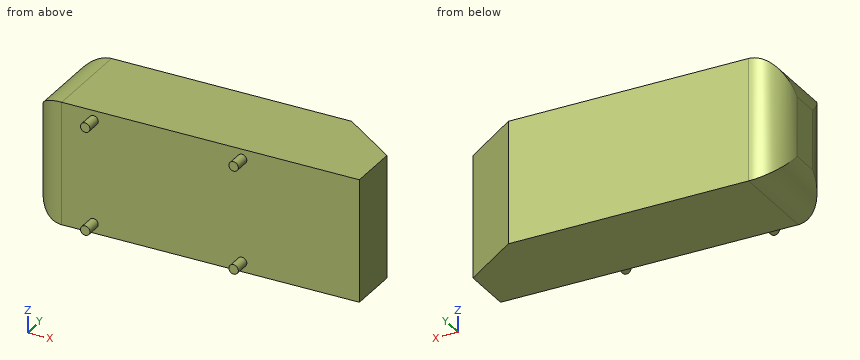
from build123d import *

# Parameters (mm, degrees)
F1_DEPTH = 194.5
F2_DEPTH = 194.5
F3_R     = 15
F5_R     = 100


with BuildPart() as f1:
    # F0 (on Top) → F1 (new body)
    with BuildSketch(Plane.XY):
        Polygon((-1043.9980842894, 48), (0, 50), (0, 210.6660311301), (-181.8517538322, 338), (-1043.9980842894, 338), (-1043.9980842894, 50), align=None)
    extrude(amount=F1_DEPTH)

    # F0 (on Top) → F2 (join)
    with BuildSketch(Plane.XY):
        Polygon((-1043.9980842894, 48), (0, 50), (0, 210.6660311301), (-181.8517538322, 338), (-1043.9980842894, 338), (-1043.9980842894, 50), align=None)
    extrude(amount=-F2_DEPTH)

    # F3 (on Front) → F4 (join, up to the next surface of F1)
    with BuildSketch(Plane.XZ):
        with Locations((-843, 163.5)):
            Circle(F3_R)
        with Locations((-843, -163.5)):
            Circle(F3_R)
        with Locations((-372, 163.5)):
            Circle(F3_R)
        with Locations((-372, -163.5)):
            Circle(F3_R)
    extrude(until=Until.NEXT, dir=(0, 1, 0))

    # F5
    f5_edges = [f1.edges().sort_by_distance(p)[0] for p in [
        (-1043.998084, 338, 0),
        (-1043.998084, 193, 194.5),
        (-1043.998084, 48, 0),
        (-1043.998084, 193, -194.5),
    ]]
    fillet(f5_edges, radius=F5_R)


solid = f1.part
CAD build for the part. Positions are in the model's coordinates, mm. Give positions to 0.01 mm unless a question says otherwise; leave off trailing zeros. Loops run counter-clockwise (first coordinate to the right, second up) from the corner with the lowest first, then second, coordinate; pieces in that order, holes last. Notation, with made-up numbers: M 85,0 L 90,0 A11 ccw 90,20 Z; hole C 53.5,19.5 d6. An arc over 180 degrees is marked long. One line per question, with ' | ' between items. Start each with the question number.
1. Saw through at A-A on z = -80. Give the cut face in (x, y), plus the area to 3 significant figures.
2. Saw through at C-C on x = -843. Give the cut face in (y, z), plus the area to 3 significant figures.
3. Probe L1, parallel to Z at x = -949.5, y = 77; L2, parallel to Y at x = -869, z = -69; L3, parallel to Y at x = -357, z = -75. List the from-to ranges inside material, lowest first. Write a range as from..to.
4. Saw through at D-D on y = 307. Give the cut face in (x, z).
5. Flat gauge pins, fed straight in: pin 1 (8 mm diameter, centred on x = -130.5, z = 62.5, fed in from -Y); pin 2 (8 mm diameter, centred on x = -581.5, z = -4.5, fed in from -Y). Where does each tip first touch, or does it go through?
6. Saw through at B-B on y = 25. Give the cut face in (x, z), plus the area to 3 significant figures.
Result sheet:
1) outline: M -1044,148.19 A100 ccw -943.81,48.19 L 0,50 L 0,210.67 L -181.85,338 L -944,338 A100 ccw -1044,238 Z | area: 286,000 mm^2
2) outline: M 0,-178.5 L 48.39,-178.5 L 48.39,-194.5 L 338,-194.5 L 338,194.5 L 48.39,194.5 L 48.39,178.5 L 0,178.5 L 0,148.5 L 48.39,148.5 L 48.39,-148.5 L 0,-148.5 Z | area: 116,000 mm^2
3) L1: z = -194.35..194.35 | L2: y = 48.34..338 | L3: y = 49.32..338
4) outline: M -1016.38,-163.5 A100 ccw -944,-194.5 L -137.58,-194.5 L -137.58,194.5 L -944,194.5 A100 ccw -1016.38,163.5 Z
5) pin 1: stops at y = 49.74 | pin 2: stops at y = 48.88
6) outline: C -843,-163.5 d30; C -843,163.5 d30; C -372,-163.5 d30; C -372,163.5 d30 | area: 2,830 mm^2
